from build123d import *

# Parameters (mm, degrees)
SKETCH1_W           = 295
SKETCH1_H           = 125
BOSS_EXTRUDE3_DEPTH = 5
SKETCH2_W           = 295
SKETCH2_H           = 115
BOSS_EXTRUDE4_DEPTH = 20
SKETCH4_W           = 140
SKETCH4_H           = 50
CUT_EXTRUDE1_DEPTH  = 17.5
SKETCH4_3_W         = 140
SKETCH4_3_H         = 50
CUT_EXTRUDE2_DEPTH  = 17.5
SKETCH7_R           = 15
CUT_EXTRUDE3_DEPTH  = 31.5


with BuildPart() as part:
    # Sketch1 → Boss-Extrude3 (new body)
    with BuildSketch(Plane(origin=(0, 0, 0), x_dir=(1, 0, 0), z_dir=(0, 1, 0))):
        with Locations((24.344660194, 23.262829884)):
            Rectangle(SKETCH1_W, SKETCH1_H)
    extrude(amount=-BOSS_EXTRUDE3_DEPTH)

    # Sketch2 → Boss-Extrude4 (add)
    with BuildSketch(Plane(origin=(0, 0, 0), x_dir=(1, 0, 0), z_dir=(0, 1, 0))):
        with Locations((24.344660194, 23.262829884)):
            Rectangle(SKETCH2_W, SKETCH2_H)
    extrude(amount=-BOSS_EXTRUDE4_DEPTH)

    # Sketch4 → Cut-Extrude1 (cut)
    with BuildSketch(Plane(origin=(0, 0, 0), x_dir=(1, 0, 0), z_dir=(0, 1, 0))):
        with Locations((-48.155339806, 50.762829884)):
            Rectangle(SKETCH4_W, SKETCH4_H)
    extrude(amount=-CUT_EXTRUDE1_DEPTH, mode=Mode.SUBTRACT)

    # Sketch4<3> → Cut-Extrude2 (cut)
    with BuildSketch(Plane(origin=(0, 0, 0), x_dir=(1, 0, 0), z_dir=(0, 1, 0))):
        with Locations((-48.155339806, 50.762829884)):
            Rectangle(SKETCH4_3_W, SKETCH4_3_H)
        with Locations((96.844660194, 50.762829884)):
            Rectangle(SKETCH4_3_W, SKETCH4_3_H)
        with Locations((96.844660194, -4.237170116)):
            Rectangle(SKETCH4_3_W, SKETCH4_3_H)
        with Locations((-48.155339806, -4.237170116)):
            Rectangle(SKETCH4_3_W, SKETCH4_3_H)
    extrude(amount=-CUT_EXTRUDE2_DEPTH, mode=Mode.SUBTRACT)

    # Sketch7 → Cut-Extrude3 (cut)
    with BuildSketch(Plane(origin=(0, -17.5, 0), x_dir=(1, 0, 0), z_dir=(0, 1, 0))):
        with Locations((-48.155339806, -4.237170116)):
            Circle(SKETCH7_R)
        with Locations((96.844660194, -4.237170116)):
            Circle(SKETCH7_R)
        with Locations((96.844660194, 50.762829884)):
            Circle(SKETCH7_R)
        with Locations((-48.155339806, 50.762829884)):
            Circle(SKETCH7_R)
    extrude(amount=-CUT_EXTRUDE3_DEPTH, mode=Mode.SUBTRACT)


solid = part.part
Here's how the part is built. I have some questions about the finished solid (model axes, mm). A direction names the side the tool comes from. Round coordinates to 2 decimals unless told otherwise and drop trailing zeros. Loops run counter-clockwise (first coordinate to the right, second up) from the corner with the lowest first, then second, coordinate; pieces in that order, holes last.
1. If we section it at D-D on z = 13: Write out the boundary of the cut face in (x, y), plus the area to 3 significant figures.
Answer list:
outline: (-123.16, -20) - (-60.33, -20) - (-60.33, -17.5) - (-118.16, -17.5) - (-118.16, 0) - (-123.16, 0) - close; (-35.98, -20) - (84.67, -20) - (84.67, -17.5) - (26.84, -17.5) - (26.84, 0) - (21.84, 0) - (21.84, -17.5) - (-35.98, -17.5) - close; (109.02, -20) - (171.84, -20) - (171.84, 0) - (166.84, 0) - (166.84, -17.5) - (109.02, -17.5) - close
area: 878 mm2
2. For P1, Ø25, axis at x = -48, z = -61.5, coming from the +Y side; P2, Ø8, axis at x = 53.5, y = -12.5, coming from the -Z side; P3, Ø2.5, axis at x = 74.5, z = 36.5, coming from the -Y side, each with a flat end and sliding along its axis, tell me the tip position at first contact or that it passes through.
Answer list:
P1: stops at y = -17.5
P2: stops at z = -80.76
P3: stops at y = -5
3. If I drill on line 1 along X through (y, z) = (-6.75, 2); line 2 along Z through (x, y) = (-40, -11.5); line 3 along Z through (x, y) = (43.5, -0.75), over which ranges is the centre line in solid material (lowest first)?
Answer list:
line 1: x = -123.16 to -118.16, 21.84 to 26.84, 166.84 to 171.84
line 2: z = -80.76 to -75.76, -25.76 to -20.76, 29.24 to 34.24
line 3: z = -85.76 to -75.76, -25.76 to -20.76, 29.24 to 39.24
4. Which directions (+Z, -Z, +X, -X, +Y, -Y) give clear straight access to the entire face, cutting with the end or side of a thin tool? Please do faces 4 (the face through (22, -5, 37)), 5 (the face through (22, -5, -83)), 6 (the face through (96, -9, 29.237)).
Answer list:
face 4: +Z, +X, -X, -Y
face 5: -Z, +X, -X, -Y
face 6: +Y
5. We'd pull the mould along X, two halves only. Please class faces 1 (the face through (-49, -9, -20.763)), 2 (the face through (-59.21, -18.73, -60.9)), 3 (the face through (22, -20, -24)): +X half, -X half, draft (parallel to the pull), parting line (faces both ways), or undercut.
Answer list:
face 1: undercut
face 2: undercut
face 3: draft
6. If we section it at C-C on z = -30.5: Write out the boundary of the cut face in (x, y).
Answer list:
outline: (-123.16, -20) - (171.84, -20) - (171.84, 0) - (166.84, 0) - (166.84, -17.5) - (26.84, -17.5) - (26.84, 0) - (21.84, 0) - (21.84, -17.5) - (-118.16, -17.5) - (-118.16, 0) - (-123.16, 0) - close
7. If we section it at B-B on x = -82: Write out the boundary of the cut face in (y, z), plus the area to 3 significant figures.
Answer list:
outline: (-20, -80.76) - (-5, -80.76) - (-5, -85.76) - (0, -85.76) - (0, -75.76) - (-17.5, -75.76) - (-17.5, -25.76) - (0, -25.76) - (0, -20.76) - (-17.5, -20.76) - (-17.5, 29.24) - (0, 29.24) - (0, 39.24) - (-5, 39.24) - (-5, 34.24) - (-20, 34.24) - close
area: 600 mm2
8. If we section it at A-A on y = -13.75: Write out the boundary of the cut face in (x, z).
Answer list:
outline: (-123.16, -80.76) - (171.84, -80.76) - (171.84, 34.24) - (-123.16, 34.24) - close; hole (-118.16, -75.76) - (21.84, -75.76) - (21.84, -25.76) - (-118.16, -25.76) - close; hole (-118.16, -20.76) - (21.84, -20.76) - (21.84, 29.24) - (-118.16, 29.24) - close; hole (26.84, -75.76) - (166.84, -75.76) - (166.84, -25.76) - (26.84, -25.76) - close; hole (26.84, -20.76) - (166.84, -20.76) - (166.84, 29.24) - (26.84, 29.24) - close
